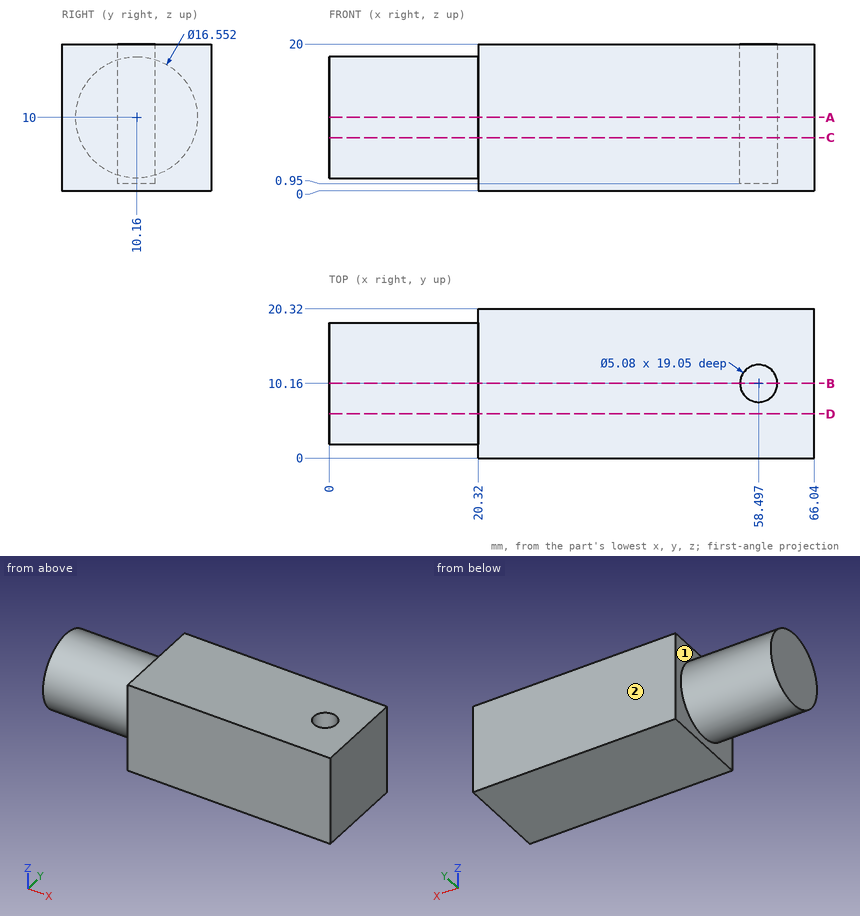
Study the drawing (mm; zero at the part's minimum x, y, z) and answer. A direction names the side the tool comes from. Coordinates: 2 decimals unless noted, no trailing zeros. Loops run counter-clockwise (first coordinate to the right, second up) from the corner with the lowest first, then second, coordinate; pieces in that order, holes last. Notation, with made-up numbers: (82, 48) -> (110, 48) arc R23 cw to (110, 78) -> close; hole circle Ø1 at (-29.5, 82). An arc over 180 degrees is marked (long way). Write each question's results on one line, items separated by ' | '. Start each with the question number.
1) Find section B-B on y = 10.16. Determine the outline of the cut face in (x, z).
2) Find section C-C on z = 7.25. Determine the outline of the cut face in (x, y) (1 decimal), then the cut area to 3 significant figures.
3) Find section D-D on y = 6. Determine the outline of the cut face in (x, z) (1 decimal), then the cut area to 3 significant figures.
4) For the marked faces 1 and 2, determine the directions among +Z, -Z, +X, -X, +Y, -Y from which every point of the face is accessible in a straight line to the end or side of a thin tool.
5) A flat-ended cylindrical pin translates along its axis: P1, Ø2.5, axis at x = 58, y = 10, coming from the +Z side. Find the tip coordinate at first contact, or state that the pin passes through.
6) Consider line 1 along X through (y, z) = (14, 18); line 2 along Y through (x, z) = (58, 9); line 3 along X through (y, z) = (11.5, 2) (1 decimal). Determine where each line is inside the solid, lowest interval first.
7) Find section A-A on z = 10. Determine the outline of the cut face in (x, y).
Response values:
1) outline: (0, 1.72) -> (20.32, 1.72) -> (20.32, 0) -> (66.04, 0) -> (66.04, 20) -> (61.04, 20) -> (61.04, 0.95) -> (55.96, 0.95) -> (55.96, 20) -> (20.32, 20) -> (20.32, 18.28) -> (0, 18.28) -> close
2) outline: (0, 2.4) -> (20.3, 2.4) -> (20.3, 0) -> (66, 0) -> (66, 20.3) -> (20.3, 20.3) -> (20.3, 18) -> (0, 18) -> close; hole circle Ø5.1 at (58.5, 10.2) | area: 1,230 mm^2
3) outline: (0, 2.8) -> (20.3, 2.8) -> (20.3, 0) -> (66, 0) -> (66, 20) -> (20.3, 20) -> (20.3, 17.2) -> (0, 17.2) -> close | area: 1,210 mm^2
4) face 1: -X | face 2: +Z, -Z, +X, -X, +Y
5) P1: stops at z = 0.95
6) line 1: x = 20.32 to 66.04 | line 2: y = 0 to 7.67, 12.65 to 20.32 | line 3: x = 0 to 56.3, 60.7 to 66
7) outline: (0, 1.88) -> (20.32, 1.88) -> (20.32, 0) -> (66.04, 0) -> (66.04, 20.32) -> (20.32, 20.32) -> (20.32, 18.44) -> (0, 18.44) -> close; hole circle Ø5.08 at (58.5, 10.16)
